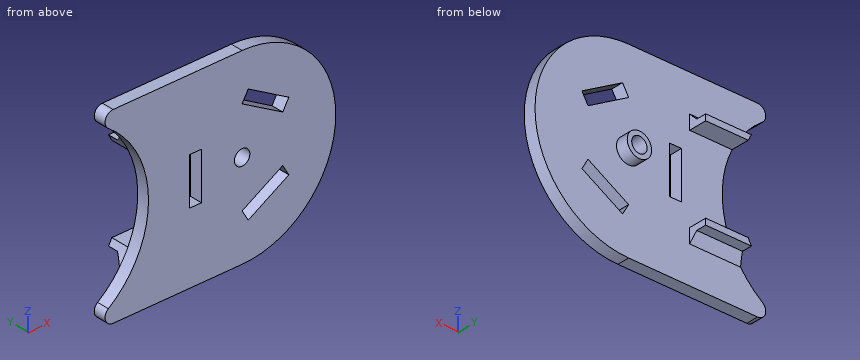
Autodesk Inventor part; units mm, degrees
ref_plane "YZ Plane" through (0, 0, 0) normal (1, 0, 0) x (0, 1, 0)
ref_plane "XZ Plane" through (0, 0, 0) normal (0, 1, 0) x (-1, 0, 0)
ref_plane "XY Plane" through (0, 0, 0) normal (0, 0, 1) x (1, 0, 0)
sketch "スケッチ1" plane through (0, 0, 0) normal (0, 1, 0) x (-1, 0, 0)
  circle A0 centre (0, 0) radius 6
  dimension "d0" = 12
extrude "押し出し1" add sketch "スケッチ1" along normal blind 1
sketch "スケッチ2" plane through (0, 1, 0) normal (0, 1, 0) x (1, 0, 0)
  circle A0 centre (0, 0) radius 3
  dimension "d3" = 6
extrude "押し出し2" add sketch "スケッチ2" along normal blind 3
sketch "スケッチ3" plane through (0, 4, 0) normal (0, 1, 0) x (1, 0, 0)
  circle A0 centre (0, 0) radius 1.9
  dimension "d6" = 3.8
extrude "押し出し3" cut sketch "スケッチ3" against normal through all
sketch "スケッチ4" plane through (0, 1, 0) normal (0, 1, 0) x (1, 0, 0)
  circle A0 centre (0, 0) radius 23.55
  circle A1 centre (-47.1, 0) radius 23.55
  line L0 (-47.1, 23.55) -> (0, 23.55)
  line L1 (0, -23.55) -> (-47.1, -23.55)
  circle A2 centre (0, 0) radius 1.9
  dimension "d11" = 47.1
extrude "押し出し4" add sketch "スケッチ4" against normal blind 3 contours A0 | A0 A1 L0 | L1 A1 A0
sketch "スケッチ5" plane through (0, -2, 0) normal (0, -1, 0) x (1, 0, 0)
  circle A0 centre (0, 0) radius 23.05
  circle A1 centre (-47.1, 0) radius 24.05
  arc A2 (0, -23.55) -> (0, 23.55) centre (0, 0) ccw
  arc A3 (-47.1, -23.55) -> (-47.1, 23.55) centre (-47.1, 0) ccw
  line L0 (0, 23.05) -> (-40.2371, 23.05)
  line L1 (0, -23.05) -> (-40.2371, -23.05)
  line L2 (30, 40) -> (-80, 40)
  line L3 (-80, 40) -> (-80, -50)
  line L4 (-80, -50) -> (30, -50)
  line L5 (30, -50) -> (30, 40)
  dimension "d14" = 0.5
  dimension "d15" = 0.5
extrude "押し出し5" cut sketch "スケッチ5" against normal through all contours A1 | L5 L4 L3 L2
fillet "フィレット1" radius 2 2 edges at (-40.2371, -0.5, 23.05) (-40.2371, -0.5, -23.05)
sketch "スケッチ6" plane through (0, -2, 0) normal (0, -1, 0) x (1, 0, 0)
  circle A0 centre (0, 0) radius 10
  line L0 (10, 5.7735) -> (10, -5.7735)
  line L1 (10, -5.7735) -> (0, -11.547)
  line L2 (0, -11.547) -> (-10, -5.7735)
  line L3 (-10, -5.7735) -> (-10, 5.7735)
  line L4 (-10, 5.7735) -> (0, 11.547)
  line L5 (0, 11.547) -> (10, 5.7735)
  line L6 (-10, -5.7735) -> (-10, 5.7735)
  line L7 (-10, 5.7735) -> (-13, 5.7735)
  line L8 (-13, 5.7735) -> (-13, -5.7735)
  line L9 (-13, -5.7735) -> (-10, -5.7735)
  line L10 (0, 11.547) -> (10, 5.7735)
  line L11 (10, 5.7735) -> (11.5, 8.3716)
  line L12 (11.5, 8.3716) -> (1.5, 14.1451)
  line L13 (1.5, 14.1451) -> (0, 11.547)
  line L14 (10, -5.7735) -> (0, -11.547)
  line L15 (0, -11.547) -> (1.5, -14.1451)
  line L16 (1.5, -14.1451) -> (11.5, -8.3716)
  line L17 (11.5, -8.3716) -> (10, -5.7735)
  point P0 (10, -5.7735)
  dimension "d19" = 20
  dimension "d20" = 3
  dimension "d21" = 3
  dimension "d22" = 3
extrude "押し出し6" cut sketch "スケッチ6" against normal through all contours L5 L13 L12 L11 | L1 L17 L16 L15 | L3 L9 L8 L7
sketch "スケッチ7" plane through (0, 1, 0) normal (0, 1, 0) x (1, 0, 0)
  line L0 (0, 10.5) -> (-45, 10.5)
  line L1 (-45, 10.5) -> (-45, -10.5)
  line L2 (-45, -10.5) -> (0, -10.5)
  line L3 (0, -10.5) -> (0, 10.5)
  line L4 (-15, 10.5) -> (-45, 10.5)
  line L5 (-45, 10.5) -> (-45, 12)
  line L6 (-45, 12) -> (-15, 12)
  line L7 (-15, 12) -> (-15, 10.5)
  line L8 (-15, -10.5) -> (-45, -10.5)
  line L9 (-45, -10.5) -> (-45, -12)
  line L10 (-45, -12) -> (-15, -12)
  line L11 (-15, -12) -> (-15, -10.5)
  arc A0 (-32.9322, -19.4339) -> (-32.9322, 19.4339) centre (-47.1, 0) ccw
  point P0 (0, 0)
  point P1 (0, 0)
  point P2 (-25.4632, -10.5)
  point P3 (-26.2577, -12)
  point P4 (-26.2577, 12)
  point P5 (-25.4632, 10.5)
  dimension "d25" = 21
  dimension "d26" = 15
  dimension "d27" = 1.5
  dimension "d28" = 1.5
extrude "押し出し7" add sketch "スケッチ7" along normal blind 4.5 contours L0 A0 L6 L7 | L11 L10 A0 L2
chamfer "面取り1" distance 2 angle 45 2 edges at (-20.6288, 1, 12) (-20.6288, 1, -12)
properties part number "ベルト_bush_upper"
For this review, take the finished solid that the model builds, in its own axes (mm). Give positions to 0.01 mm unless a question says otherwise; leave off trailing zeros. Loops run counter-clockwise (first coordinate to the right, second up) from the corner with the lowest first, then second, coordinate; pieces in that order, holes last. Notation, with made-up numbers: M 81.5,3.5 L 135.5,3.5 A17 cw 135.5,36.5 Z; hole C -2,25.25 d2. An arc over 180 degrees is marked long. One line per item, written item: value. Start each with the question number.
Q1. Clearance check with flat-ended pins moving along their axes: pin 1 Ø1.3 at (x, y) = (-19, 3.5) entering from -Z; pin 2 Ø0.8 at (x, y) = (-18.5, 5) entering from -Z; pin 3 Ø1 at (y, z) = (4.5, 12) entering from +X. State where each tip first meets the part, or that it passes through.
Q2. For L1, parallel to X at y = 0.2, z = 0; L2, parallel to Z at x = -21, y = 4.75; L3, parallel to Z at x = 2, y = -1.5, list the stretches that pass through material, from the lowest coordinate up.
Q3. Add section D-D (x = -1). Give the boundary of the cut face in (y, z).
Q4. Add section C-C (z = 0). Give the boundary of the cut face in (x, y).
Q5. Add section A-A (y = 1.75). Give the boundary of the cut face in (x, z), and give its area (3 significant figures).
Q6. Add section B-B (x = -19.5). Give the boundary of the cut face in (y, z).
Reply:
1. pin 1: z = -12.15
1. pin 2: z = -12
1. pin 3: x = -15
2. L1: -23.05 to -13, -10 to -1.9, 1.9 to 23.05
2. L2: -12 to -10.5, 10.5 to 12
2. L3: -22.96 to -13.86, -10.39 to 10.39, 13.86 to 22.96
3. outline: M -2,-23.05 L 1,-23.05 L 1,-2.83 L 4,-2.83 L 4,-1.62 L -2,-1.62 Z; M -2,1.62 L 4,1.62 L 4,2.83 L 1,2.83 L 1,23.05 L -2,23.05 Z
4. outline: M -23.05,-2 L -13,-2 L -13,1 L -23.05,1 Z; M -10,-2 L -1.9,-2 L -1.9,4 L -3,4 L -3,1 L -10,1 Z; M 1.9,-2 L 23.05,-2 L 23.05,1 L 3,1 L 3,4 L 1.9,4 Z
5. outline: M -27.03,-13.25 L -15,-13.25 L -15,-10.5 L -25.46,-10.5 A24.05 cw Z; M -27.03,13.25 A24.05 cw -25.46,10.5 L -15,10.5 L -15,13.25 Z; C 0,0 d6; hole C 0,0 d3.8
5. area: 78.6 mm²
6. outline: M -2,-23.05 L 1,-23.05 L 1,-14 L 3,-12 L 5.5,-12 L 5.5,-10.5 L 1,-10.5 L 1,10.5 L 5.5,10.5 L 5.5,12 L 3,12 L 1,14 L 1,23.05 L -2,23.05 Z
